The model under review builds one solid part; all positions refer to its coordinate system, in mm. Face numbers are marked on the shaded views. A direction names the side the tool comes from. Coordinates: 2 decimals unless noted, no trailing zeros. Write each loop counter-clockwise with the first axis right and the second up, starting at its lowest first coordinate (ties: lowest second). Pieces come first, ordered by that corner, then holes.
```python
from build123d import *

# Parameters (mm, degrees)
BOSS_EXTRUDE1_DEPTH = 30
SKETCH2_W           = 42.5
SKETCH2_H           = 42.5
SKETCH2_W_2         = 5.2
SKETCH2_H_2         = 2.957646667
CUT_EXTRUDE1_DEPTH  = 21.27


with BuildPart() as part:
    # Sketch1 → Boss-Extrude1 (new body)
    with BuildSketch(Plane.XY):
        with BuildLine():
            Line((30.787284994, 71.307646667), (-30.787284994, 71.307646667))
            add(Edge.make_bspline(
                [(-30.787284994, 71.307646667), (-18.71151784, 42.368167262), (-24.982996832, 11.493470723)],
                knots=[0, 0, 0, 1, 1, 1], degree=2))
            ThreePointArc((-24.982996832, 11.493470723), (0, -27.5), (24.982996832, 11.493470723))
            add(Edge.make_bspline(
                [(30.787284994, 71.307646667), (18.71151784, 42.368167262), (24.982996832, 11.493470723)],
                knots=[0, 0, 0, 1, 1, 1], degree=2))
        make_face()
    extrude(amount=BOSS_EXTRUDE1_DEPTH)

    # Sketch2 → Cut-Extrude1 (cut)
    with BuildSketch(Plane.XY):
        with Locations((0, 45)):
            Rectangle(SKETCH2_W, SKETCH2_H)
        Polygon((-11.6, 66.25), (11.6, 66.25), (11.6, 68.35), (2.6, 68.35), (-2.6, 68.35), (-11.6, 68.35), align=None)
        with Locations((0, 69.828823333)):
            Rectangle(SKETCH2_W_2, SKETCH2_H_2)
    extrude(amount=CUT_EXTRUDE1_DEPTH, mode=Mode.SUBTRACT)


solid = part.part
```
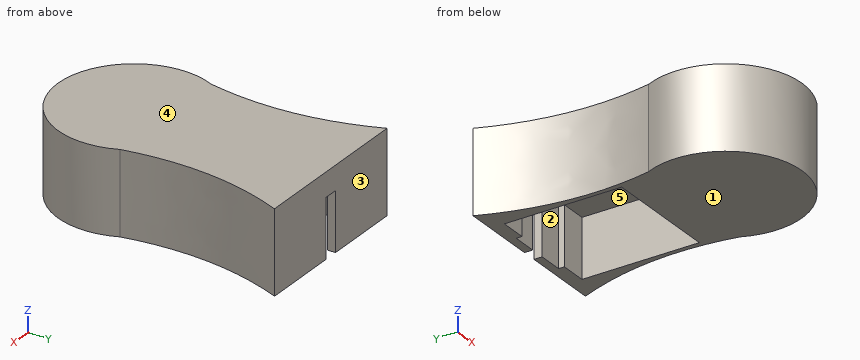
Item 1: Take a section at C-C, the plane x = 16.5. Write out the cut boundary in (y, z), plus the area to 3 significant figures.
Solved:
outline: (-22, 0) - (23.75, 0) - (23.75, 21.27) - (66.25, 21.27) - (66.25, 0) - (71.31, 0) - (71.31, 30) - (-22, 30) - close
area: 1,900 mm2
Item 2: For pin 1 (6.5 mm diameter, centred on y = 39, z = 7.5, fed in from +X); pin 2 (1.5 mm diameter, centred on y = 70.5, z = 14.5, fed in from +X); pin 3 (0.6 mm diameter, centred on y = 67, z = 7.5, fed in from -X), all flat-tipped, find the tip position at first contact; note any pin that passes through.
Solved:
pin 1: stops at x = 23.33
pin 2: stops at x = 30.76
pin 3: stops at x = -29.21
Item 3: To check wall thickness, follow line 1 along Z through (x, y) = (-20.5, 24); line 2 along Y through (x, z) = (0.5, 19); line 3 along X through (y, z) = (32.5, 29.5). State the ranges of each line that lie inside material, in increasing order.
Solved:
line 1: z = 21.27 to 30
line 2: y = -27.5 to 23.75
line 3: x = -22.84 to 22.84
Item 4: Mouldability with a two-part tool opening along Y and no side actions: class the marked faces 3, 4 and 5 as pulls with the +Y half, pulls with the -Y half, needs draft (parallel to the pull), parting line crosses it, or undercut.
Solved:
face 3: pulls with the +Y half
face 4: needs draft
face 5: undercut
Item 5: Take a section at B-B, the plane y = 0. Write out the cut boundary in (x, z), plus the area to 3 significant figures.
Solved:
outline: (-27.5, 0) - (27.5, 0) - (27.5, 30) - (-27.5, 30) - close
area: 1,650 mm2
Item 6: Take a section at A-A, the plane x = 0. Write out the cut boundary in (y, z).
Solved:
outline: (-27.5, 0) - (23.75, 0) - (23.75, 21.27) - (71.31, 21.27) - (71.31, 30) - (-27.5, 30) - close
Item 7: Machinability: for the marked faces 1 and 2, which of the approach directions +Z, -Z, +X, -X, +Y, -Y give a long, thin tool a straight path to every point of the face, cutting with its end or side? Answer none if there is none.
Solved:
face 1: -Z, +X, -X, +Y, -Y
face 2: -Z
Item 8: Take a section at D-D, the plane x = -9. Write out the cut boundary in (y, z), plus the area to 3 significant figures.
Solved:
outline: (-25.99, 0) - (23.75, 0) - (23.75, 21.27) - (68.35, 21.27) - (68.35, 0) - (71.31, 0) - (71.31, 30) - (-25.99, 30) - close
area: 1,970 mm2
